The model under review builds one solid part; all positions refer to its coordinate system, in mm. Face numbers are marked on the shaded views. A direction names the side the tool comes from. Give positions to 0.01 mm unless a question says otherwise; leave off trailing zeros. Write each loop counter-clockwise with the first axis right and the second up, starting at its lowest first coordinate (ties: lowest second). Pieces come first, ordered by that corner, then holes. Notation, with made-up numbers: (80, 51.5) -> (125, 51.5) arc R16 ccw to (125, 74.5) -> close; hole circle Ø2 at (-35, 62.25). An arc over 180 degrees is marked (long way). Use CSV: the item, a comma, the result in double quotes.
```python
from build123d import *

# Parameters (mm, degrees)
F0_W     = 10
F0_H     = 10
F0_W_2   = 8
F0_H_2   = 8
F1_DEPTH = 63
F2_R     = 1.5
F3_DEPTH = 25
F4_R     = 1.5
F5_DEPTH = 25


with BuildPart() as f1:
    # F0 (on Top) → F1 (new body)
    with BuildSketch(Plane.XY):
        Rectangle(F0_W, F0_H)
        Rectangle(F0_W_2, F0_H_2, mode=Mode.SUBTRACT)
    extrude(amount=F1_DEPTH)

    # F2 (on face) → F3 (cut)
    with BuildSketch(Plane.XZ.offset(5)):
        with Locations((0, 5)):
            Circle(F2_R)
        with Locations((0, 58)):
            Circle(F2_R)
    extrude(amount=-F3_DEPTH, mode=Mode.SUBTRACT)

    # F4 (on face) → F5 (cut)
    with BuildSketch(Plane.YZ.offset(5)):
        with Locations((0, 48)):
            Circle(F4_R)
        with Locations((0, 15)):
            Circle(F4_R)
    extrude(amount=-F5_DEPTH, mode=Mode.SUBTRACT)


solid = f1.part
```
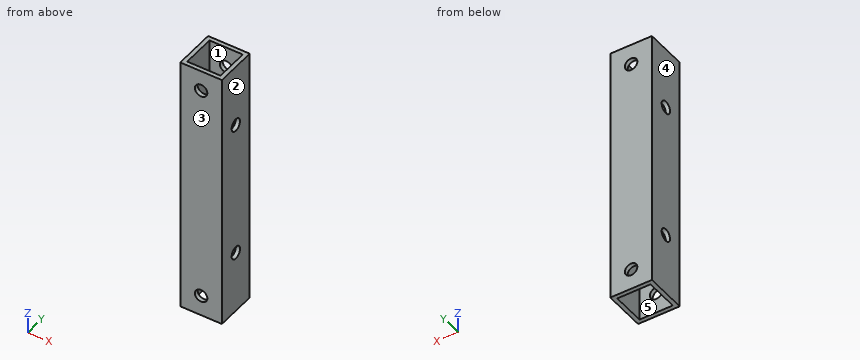
Q1. To check wall thickness, follow probe 1 along Z at (x, y) = (4.5, 0); probe 2 along Z at (x, y) = (0, 4.45); probe 3 along Y at (x, z) = (-1.5, 48.5). State the ranges of each line that lie inside material, in increasing order.
Derived:
probe 1,"z = 0 to 13.5, 16.5 to 46.5, 49.5 to 63"
probe 2,"z = 0 to 3.5, 6.5 to 56.5, 59.5 to 63"
probe 3,"y = -5 to -4, 4 to 5"
Q2. Machinability: for the marked faces 1 and 2, which of the approach directions +Z, -Z, +X, -X, +Y, -Y give a long, thin tool a straight path to every point of the face, cutting with its end or side? Answer none if there is none.
Derived:
face 1,"+Z, -Z"
face 2,"+Z, -Z, +X, +Y, -Y"
Q3. The part is to be moulded in two halves that separate along X. For the marked faces 3, 4 and 5, say which applies: pulls with the +X half, pulls with the -X half, needs draft (parallel to the pull), parting line crosses it, or undercut.
Derived:
face 3,"needs draft"
face 4,"pulls with the -X half"
face 5,"undercut"
Q4. Consider section A-A (x = 2.5). Write out the cut boundary in (y, z), then the cut area to 3 significant figures.
Derived:
outline,"(-5, 0) -> (-4, 0) -> (-4, 63) -> (-5, 63) -> close; (4, 0) -> (5, 0) -> (5, 63) -> (4, 63) -> close"
area,"126 mm2"
Q5. Consider section B-B (y = 0). Write out the cut boundary in (x, z).
Derived:
outline,"(-5, 0) -> (-4, 0) -> (-4, 13.5) -> (-5, 13.5) -> close; (-5, 16.5) -> (-4, 16.5) -> (-4, 46.5) -> (-5, 46.5) -> close; (-5, 49.5) -> (-4, 49.5) -> (-4, 63) -> (-5, 63) -> close; (4, 0) -> (5, 0) -> (5, 13.5) -> (4, 13.5) -> close; (4, 16.5) -> (5, 16.5) -> (5, 46.5) -> (4, 46.5) -> close; (4, 49.5) -> (5, 49.5) -> (5, 63) -> (4, 63) -> close"
Q6. Consider section C-C (z = 48). Write out the cut boundary in (x, y).
Derived:
outline,"(-5, -5) -> (5, -5) -> (5, -1.5) -> (4, -1.5) -> (4, -4) -> (-4, -4) -> (-4, -1.5) -> (-5, -1.5) -> close; (-5, 1.5) -> (-4, 1.5) -> (-4, 4) -> (4, 4) -> (4, 1.5) -> (5, 1.5) -> (5, 5) -> (-5, 5) -> close"
Q7. Insertion check: pin 1 (1.8 mm diameter, centred on y = 0, z = 48, fed in from -X). The pin has a flat end and moves straight along its axis. Give the tip position at first contact, or say it passes through.
Derived:
pin 1,"passes through"
Q8. Consider section D-D (x = 0). Write out the cut boundary in (y, z).
Derived:
outline,"(-5, 0) -> (-4, 0) -> (-4, 3.5) -> (-5, 3.5) -> close; (-5, 6.5) -> (-4, 6.5) -> (-4, 56.5) -> (-5, 56.5) -> close; (-5, 59.5) -> (-4, 59.5) -> (-4, 63) -> (-5, 63) -> close; (4, 0) -> (5, 0) -> (5, 3.5) -> (4, 3.5) -> close; (4, 6.5) -> (5, 6.5) -> (5, 56.5) -> (4, 56.5) -> close; (4, 59.5) -> (5, 59.5) -> (5, 63) -> (4, 63) -> close"
